```python
from build123d import *

# Parameters (mm, degrees)
SKETCH1_R                   = 15.875
SKETCH1_R_2                 = 11.7475
BOSS_EXTRUDE1_DEPTH         = 101.6
F_1_4_START                 = 10
F_1_4_CLEARANCE_SLOT1_DEPTH = 7
CUT_EXTRUDE1_REACH          = 106.051
CUT_EXTRUDE1_END_RADIUS     = 15.875
CUT_EXTRUDE2_DEPTH          = 105.050907141
CUT_EXTRUDE2_DEPTH_BACK     = 105.050907141
SKETCH5_R                   = 3.3655
CUT_EXTRUDE3_DEPTH          = 105.050907141
CUT_EXTRUDE3_DEPTH_BACK     = 105.050907141
SKETCH6_R                   = 3.3655


with BuildPart() as part:
    # Sketch1 → Boss-Extrude1 (new body)
    with BuildSketch(Plane.XY):
        Circle(SKETCH1_R)
        Circle(SKETCH1_R_2, mode=Mode.SUBTRACT)
    extrude(amount=BOSS_EXTRUDE1_DEPTH)

    # 1/4 Clearance Slot1: read off the stored shape, not the designer's step
    # 1/4 Clearance Slot1 outline → 1/4 Clearance Slot1 (cut)
    with BuildSketch(Plane(origin=(0, 0, 0), x_dir=(1, 0, 0), z_dir=(0, 1, 0)).offset(F_1_4_START)):
        with BuildLine():
            Line((3.3782, -88.6968), (3.3782, -25.6032))
            ThreePointArc((3.3782, -25.6032), (0, -22.225), (-3.3782, -25.6032))
            Line((-3.3782, -25.6032), (-3.3782, -88.6968))
            ThreePointArc((-3.3782, -88.6968), (0, -92.075), (3.3782, -88.6968))
        make_face()
    extrude(amount=F_1_4_CLEARANCE_SLOT1_DEPTH, mode=Mode.SUBTRACT)

    # Cut-Extrude1: up to this cylinder (the profile starts inside it)
    cut_extrude1_end = Plane(origin=(0, 0, 57.15), z_dir=(0, 0, -1)) * Cylinder(CUT_EXTRUDE1_END_RADIUS, 244.852, mode=Mode.PRIVATE)
    # Sketch4 → Cut-Extrude1 (cut, up to the surface)
    with BuildSketch(Plane(origin=(0, 0, 0), x_dir=(1, 0, 0), z_dir=(0, 1, 0)), mode=Mode.PRIVATE) as cut_extrude1_sk1:
        with BuildLine():
            Line((-3.3782, -88.6968), (-3.3782, -25.6032))
            ThreePointArc((-3.3782, -25.6032), (0, -22.225), (3.3782, -25.6032))
            Line((3.3782, -25.6032), (3.3782, -88.6968))
            ThreePointArc((3.3782, -88.6968), (0, -92.075), (-3.3782, -88.6968))
        make_face()
    cut_extrude1_tool1 = extrude(cut_extrude1_sk1.sketch, amount=-CUT_EXTRUDE1_REACH, mode=Mode.PRIVATE) & cut_extrude1_end
    add(cut_extrude1_tool1.solids().sort_by_distance((0, 0, 57.15))[0], mode=Mode.SUBTRACT)

    # Sketch5 → Cut-Extrude2 (cut, two sides: drawn at the far end of the back side and taken through both)
    with BuildSketch(Plane(origin=(0, 0, 0), x_dir=(1, 0, 0), z_dir=(0, 1, 0)).offset(-CUT_EXTRUDE2_DEPTH_BACK)):
        with Locations(Location((0, -9.525, 0), (0, 0, 270))):
            Circle(SKETCH5_R)
    extrude(amount=CUT_EXTRUDE2_DEPTH + CUT_EXTRUDE2_DEPTH_BACK, mode=Mode.SUBTRACT)

    # Sketch6 → Cut-Extrude3 (cut, two sides: drawn at the far end of the back side and taken through both)
    with BuildSketch(Plane(origin=(0, 0, 0), x_dir=(0, 0, -1), z_dir=(1, 0, 0)).offset(-CUT_EXTRUDE3_DEPTH_BACK)):
        with Locations((-9.525, 0)):
            Circle(SKETCH6_R)
    extrude(amount=CUT_EXTRUDE3_DEPTH + CUT_EXTRUDE3_DEPTH_BACK, mode=Mode.SUBTRACT)


solid = part.part
```
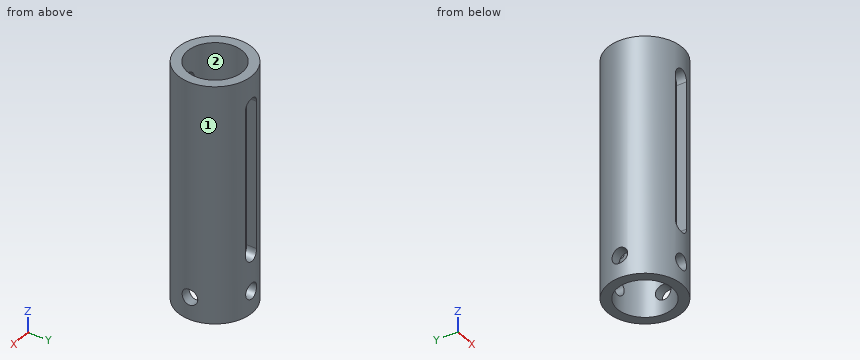
The model under review builds one solid part; all positions refer to its coordinate system, in mm. Face numbers are marked on the shaded views. Round coordinates to 2 decimals unless told otherwise and drop trailing zeros. Write each loop counter-clockwise with the first axis right and the second up, starting at its lowest first coordinate (ties: lowest second). Pieces come first, ordered by that corner, then holes. Notation, with made-up numbers: (86, 17) - (105, 17) arc R23 cw to (105, 48) - close; hole circle Ø2 at (71, -23). An arc over 180 degrees is marked (long way). Use one line per item in the form item = value.
Q1. Draft analysis for pull direction X (two halves, no side actions). For the marked faces 1 and 2, state which applies: +X half, -X half, draft (parallel to the pull), parting line (faces both ways), or undercut.
Answer key:
face_1 = parting line
face_2 = undercut
Q2. Consider section D-D (y = 8.5). State the section outline as (x, z) points.
Answer key:
outline = (-13.41, 0) - (-8.11, 0) - (-8.11, 101.6) - (-13.41, 101.6) - close; (8.11, 0) - (13.41, 0) - (13.41, 101.6) - (8.11, 101.6) - close
Q3. Consider section C-C (y = 0). State the section outline as (x, z) points (1 decimal).
Answer key:
outline = (-15.9, 0) - (-11.7, 0) - (-11.7, 6.2) - (-15.9, 6.2) - close; (-15.9, 12.9) - (-11.7, 12.9) - (-11.7, 101.6) - (-15.9, 101.6) - close; (11.7, 0) - (15.9, 0) - (15.9, 6.2) - (11.7, 6.2) - close; (11.7, 12.9) - (15.9, 12.9) - (15.9, 101.6) - (11.7, 101.6) - close
Q4. Insertion check: pin 1 Ø1.3 at (y, z) = (-13, 63.5) entering from +X; pin 2 Ø1.3 at (y, z) = (13.5, 66) entering from -X; pin 3 Ø1 at (y, z) = (-3, 17.5) entering from -X; pin 4 Ø6 at (x, z) = (2, 19.5) entering from -Y (3 decimals). Each pin has a flat end and moves straight along its axis. Give the tip position at first contact, or say it passes through.
Answer key:
pin_1 = 9.97
pin_2 = -9.32
pin_3 = -15.68
pin_4 = -15.875
Q5. For line 1 (X direction, y = 0, z = 45) (1 decimal); line 2 (Y direction, x = -7, z = 88); line 3 (X direction, y = 3.5, z = 55.5), list the stretches that pass through material, from the lowest coordinate up. Write a range as [from, to].
Answer key:
line_1 = [-15.9, -11.7], [11.7, 15.9]
line_2 = [-14.25, -9.43], [9.43, 14.25]
line_3 = [-15.48, -11.21], [11.21, 15.48]
Q6. Consider section B-B (x = 0). State the section outline as (y, z) points (1 decimal), and give its area (3 significant figures).
Answer key:
outline = (-15.9, 0) - (-11.7, 0) - (-11.7, 6.2) - (-15.9, 6.2) - close; (-15.9, 12.9) - (-11.7, 12.9) - (-11.7, 22.2) - (-15.9, 22.2) - close; (-15.9, 92.1) - (-11.7, 92.1) - (-11.7, 101.6) - (-15.9, 101.6) - close; (11.7, 0) - (15.9, 0) - (15.9, 6.2) - (11.7, 6.2) - close; (11.7, 12.9) - (15.9, 12.9) - (15.9, 22.2) - (11.7, 22.2) - close; (11.7, 92.1) - (15.9, 92.1) - (15.9, 101.6) - (11.7, 101.6) - close
area = 207 mm2
